For this review, take the finished solid that the model builds, in its own axes (mm). Face numbers are marked on the shaded views. A direction names the side the tool comes from. Round coordinates to 2 decimals unless told otherwise and drop trailing zeros. Write each loop counter-clockwise with the first axis right and the second up, starting at its lowest first coordinate (ties: lowest second). Pieces come first, ordered by that corner, then holes. Notation, with made-up numbers: M 3,53 L 40,53 A19 ccw 40,63 Z; hole C 65.25,-14.5 d7. An arc over 180 degrees is marked long. Answer in a Markdown table with one row per item.
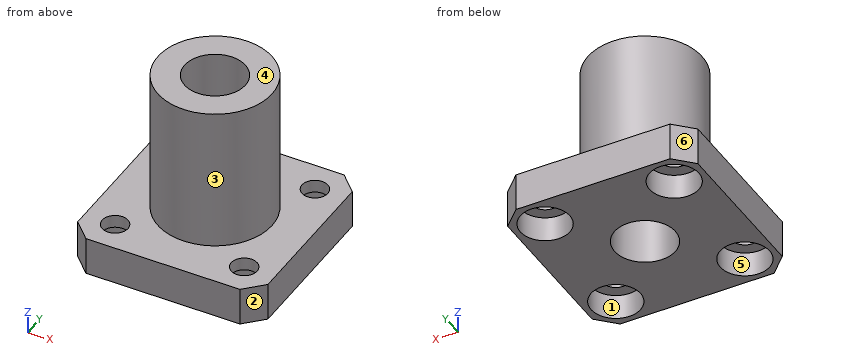
```python
from build123d import *

# Parameters (mm, degrees)
F0_W     = 25
F0_H     = 25
F0_R     = 1.7
F0_R_2   = 7.5
F0_R_3   = 4
F1_DEPTH = 3.3
F2_DEPTH = 1.7
F3_R     = 7.5
F3_R_2   = 4
F4_DEPTH = 19
F6_DEPTH = 25
F7_R     = 3.25
F7_R_2   = 1.7
F8_DEPTH = 3.3


# Not quite as in the source:
# - a feature names something its author has since deleted; it is built from what else it names


with BuildPart() as f1:
    # F0 (on Top) → F1 (new body)
    with BuildSketch(Plane.XY):
        Rectangle(F0_W, F0_H)
        with Locations((-8.4852813742, -8.4852813742)):
            Circle(F0_R, mode=Mode.SUBTRACT)
        with Locations((8.4852813742, -8.4852813742)):
            Circle(F0_R, mode=Mode.SUBTRACT)
        with Locations((-8.4852813742, 8.4852813742)):
            Circle(F0_R, mode=Mode.SUBTRACT)
        Circle(F0_R_2, mode=Mode.SUBTRACT)
        with Locations((8.4852813742, 8.4852813742)):
            Circle(F0_R, mode=Mode.SUBTRACT)
        Circle(F0_R_2)
        Circle(F0_R_3, mode=Mode.SUBTRACT)
    extrude(amount=-F1_DEPTH)

    # F0 (on Top) → F2 (join)
    with BuildSketch(Plane.XY):
        Rectangle(F0_W, F0_H)
        with Locations((-8.4852813742, -8.4852813742)):
            Circle(F0_R, mode=Mode.SUBTRACT)
        with Locations((8.4852813742, -8.4852813742)):
            Circle(F0_R, mode=Mode.SUBTRACT)
        with Locations((-8.4852813742, 8.4852813742)):
            Circle(F0_R, mode=Mode.SUBTRACT)
        Circle(F0_R_2, mode=Mode.SUBTRACT)
        with Locations((8.4852813742, 8.4852813742)):
            Circle(F0_R, mode=Mode.SUBTRACT)
        Circle(F0_R_2)
        Circle(F0_R_3, mode=Mode.SUBTRACT)
    extrude(amount=F2_DEPTH)

    # F3 (on face) → F4 (join)
    with BuildSketch(Plane.XY.offset(1.7)):
        Circle(F3_R)
        Circle(F3_R_2, mode=Mode.SUBTRACT)
    extrude(amount=F4_DEPTH)

    # F5 (on face) → F6 (cut)
    with BuildSketch(Plane.XY.offset(1.7)):
        Polygon((-12.5, 12.5), (-12.5, 10.127416998), (-10.127416998, 12.5), align=None)
        Polygon((-10.127416998, -12.5), (-12.5, -10.127416998), (-12.5, -12.5), align=None)
        Polygon((12.5, -10.127416998), (10.127416998, -12.5), (12.5, -12.5), align=None)
        Polygon((12.5, 12.5), (10.127416998, 12.5), (12.5, 10.127416998), align=None)
    extrude(amount=-F6_DEPTH, mode=Mode.SUBTRACT)

    # F7 (on face) → F8 (cut)
    with BuildSketch(Plane(origin=(0, 0, -3.3), x_dir=(1, 0, 0), z_dir=(0, 0, -1))):
        with Locations((-8.4852813742, 8.4852813742)):
            Circle(F7_R)
        with Locations((-8.4852813742, 8.4852813742)):
            Circle(F7_R_2, mode=Mode.SUBTRACT)
        with Locations((8.4852813742, 8.4852813742)):
            Circle(F7_R)
        with Locations((8.4852813742, 8.4852813742)):
            Circle(F7_R_2, mode=Mode.SUBTRACT)
        with Locations((-8.4852813742, -8.4852813742)):
            Circle(F7_R)
        with Locations((-8.4852813742, -8.4852813742)):
            Circle(F7_R_2, mode=Mode.SUBTRACT)
        with Locations((8.4852813742, -8.4852813742)):
            Circle(F7_R)
        with Locations((8.4852813742, -8.4852813742)):
            Circle(F7_R_2, mode=Mode.SUBTRACT)
    extrude(amount=-F8_DEPTH, mode=Mode.SUBTRACT)


solid = f1.part
```
Q1. Machinability: for the marked faces 1, 2 and 3, which of the approach directions +Z, -Z, +X, -X, +Y, -Y give a long, thin tool a straight path to every point of the face, cutting with its end or side? Answer none if there is none.
Found:
| item | result |
|---|---|
| face 1 | -Z |
| face 2 | +Z, -Z, +X, -Y |
| face 3 | +Z |
Q2. Insertion check: P1, Ø5, axis at x = 8.49, y = 8.49, coming from the +Z side; P2, Ø10, axis at x = 1.5, z = 9, coming from the +Y side; P3, Ø8, axis at y = -6.5, z = 14.5, coming from the -X side; P4, Ø2.5, axis at x = 8.49, y = -8.49, coming from the +Z side. Each pin has a flat end and moves straight along its axis. Give the tip position at first contact, or say it passes through.
Found:
| item | result |
|---|---|
| P1 | z = 1.7 |
| P2 | y = 7.5 |
| P3 | x = -7.07 |
| P4 | through |
Q3. For probe 1 along Z at (x, y) = (7, 4.25); probe 2 along X at (y, z) = (-0.5, -0.5); probe 3 along Y at (x, z) = (2.75, 19.25), list the stretches that pass through material, from the lowest coordinate up.
Found:
| item | result |
|---|---|
| probe 1 | -3.3 to 1.7 |
| probe 2 | -12.5 to -3.97, 3.97 to 12.5 |
| probe 3 | -6.98 to -2.9, 2.9 to 6.98 |
Q4. Take a section at D-D (z = 14.75). State the section outline as (x, y) points, then the cut area to 3 significant figures.
Found:
| item | result |
|---|---|
| outline | C 0,0 d15; hole C 0,0 d8 |
| area | 126 mm² |
Q5. Take a section at A-A (y = 0). State the section outline as (x, z) points, then the cut area to 3 significant figures.
Found:
| item | result |
|---|---|
| outline | M -12.5,-3.3 L -4,-3.3 L -4,20.7 L -7.5,20.7 L -7.5,1.7 L -12.5,1.7 Z; M 4,-3.3 L 12.5,-3.3 L 12.5,1.7 L 7.5,1.7 L 7.5,20.7 L 4,20.7 Z |
| area | 218 mm² |
Q6. Take a section at C-C (x = -9.5). State the section outline as (y, z) points.
Found:
| item | result |
|---|---|
| outline | M -12.5,-3.3 L -11.57,-3.3 L -11.57,0 L -9.85,0 L -9.85,1.7 L -12.5,1.7 Z; M -7.12,0 L -5.4,0 L -5.4,-3.3 L 5.4,-3.3 L 5.4,0 L 7.12,0 L 7.12,1.7 L -7.12,1.7 Z; M 9.85,0 L 11.57,0 L 11.57,-3.3 L 12.5,-3.3 L 12.5,1.7 L 9.85,1.7 Z |
Q7. Mouldability with a two-part tool opening along Y and no side actions: class the marked faces 4, 5 and 6 as +Y half, -Y half, draft (parallel to the pull), parting line (faces both ways), or undercut.
Found:
| item | result |
|---|---|
| face 4 | draft |
| face 5 | undercut |
| face 6 | +Y half |
